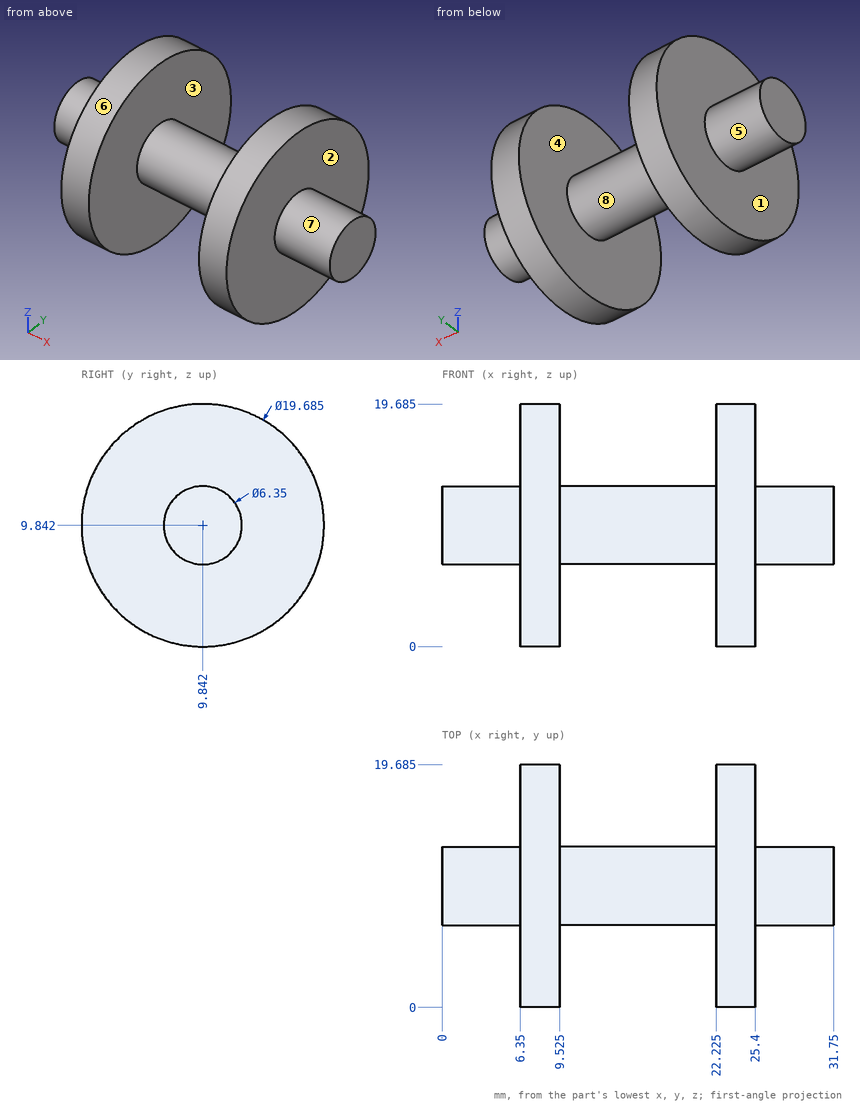
Verification items for this drawing (mm, ordinates from the low corner). A direction names the side the tool comes from. Coordinates: 2 decimals unless noted, no trailing zeros. Answer as CSV lines item,"result". Start each with the question number.
1) Gauge pin test, flat ends, axial feed: pin 1 Ø1.5 at (x, z) = (6, 5) entering from +Y (1 decimal); pin 2 Ø4 at (x, y) = (13, 14) entering from +Z; pin 3 Ø5 at (x, z) = (16, 4) entering from -Y; pin 4 Ø1.5 at (x, z) = (24.5, 17) entering from -Y. Record the tip position at first contact, or that the pin passes through.
2) Release check for a two-part mould opening along X. For the marked faces 1, 2, 3 and 4 record: released by +X, released by -X, zero draft, split by the parting line, or undercut.
3) Material ranges on L1, parallel to Z at x = 12, y = 10; L2, parallel to Z at x = 23.5, y = 3.5 (1 decimal); L3, parallel to Y at x = 5, z = 7 (1 decimal), recorded low to high. Write a range as [from, to].
4) Set-up check for the marked faces 5, 6, 7 and 8: record each of +Z, -Z, +X, -X, +Y, -Y from which the full face is reachable in a straight line by a thin tool's end or side.
Conclusion:
1,pin 1,"stops at y = 18.8"
1,pin 2,"stops at z = 12.17"
1,pin 3,"passes through"
1,pin 4,"stops at y = 2.37"
2,face 1,"released by -X"
2,face 2,"released by +X"
2,face 3,"undercut"
2,face 4,"undercut"
3,L1,"z = [6.67, 13.01]"
3,L2,"z = [2.3, 17.4]"
3,L3,"y = [8.4, 11.3]"
4,face 5,"-X"
4,face 6,"+X, -X"
4,face 7,"+X"
4,face 8,"none"
